Part model, mm, in its own coordinate system. A direction names the side the tool comes from. Round coordinates to 2 decimals unless told otherwise and drop trailing zeros. Loops run counter-clockwise (first coordinate to the right, second up) from the corner with the lowest first, then second, coordinate; pieces in that order, holes last. Notation, with made-up numbers: (-13.5, 86) -> (38.5, 86) arc R7 cw to (38.5, 98) -> close; hole circle Ø7 at (67.5, -32.5). An arc over 180 degrees is marked (long way). Answer as a JSON object with one key per item and string values. Group by question number.
from build123d import *

# Parameters (mm, degrees)
SKETCH1_W      = 50.1
SKETCH1_H      = 28.1
SKETCH1_R      = 1.7
EXTRUDE1_DEPTH = 1.54
SKETCH2_W      = 2.56
SKETCH2_H      = 15.1
SKETCH2_W_2    = 7.7
SKETCH2_H_2    = 5.4
EXTRUDE3_DEPTH = 8.4
SKETCH3_W      = 5.9
SKETCH3_H      = 7.94
EXTRUDE4_DEPTH = 5.15


with BuildPart() as part:
    # Sketch1 → Extrude1 (new body)
    with BuildSketch(Plane(origin=(0, 0, 0), x_dir=(1, 0, 0), z_dir=(0, 1, 0))):
        with Locations((-74.07266419, 15.871623192)):
            Rectangle(SKETCH1_W, SKETCH1_H)
        with Locations(Location((-96.42266419, 27.221623192, 0), (0, 0, 270))):
            Circle(SKETCH1_R, mode=Mode.SUBTRACT)
        with Locations(Location((-51.72266419, 27.221623192, 0), (0, 0, 90))):
            Circle(SKETCH1_R, mode=Mode.SUBTRACT)
        with Locations(Location((-51.72266419, 4.521623192, 0), (0, 0, 270))):
            Circle(SKETCH1_R, mode=Mode.SUBTRACT)
        with Locations(Location((-96.42266419, 4.521623192, 0), (0, 0, 90))):
            Circle(SKETCH1_R, mode=Mode.SUBTRACT)
    extrude(amount=EXTRUDE1_DEPTH)

    # Sketch2 → Extrude3 (add)
    with BuildSketch(Plane(origin=(0, 1.54, 0), x_dir=(1, 0, 0), z_dir=(0, 1, 0))):
        with Locations((-50.30266419, 15.871623192)):
            Rectangle(SKETCH2_W, SKETCH2_H)
        with Locations((-70.52266419, 4.521623192)):
            Rectangle(SKETCH2_W_2, SKETCH2_H_2)
    extrude(amount=EXTRUDE3_DEPTH)

    # Sketch3 → Extrude4 (add)
    with BuildSketch(Plane(origin=(0, 1.54, 0), x_dir=(1, 0, 0), z_dir=(0, 1, 0))):
        with Locations((-96.17266419, 19.101623192)):
            Rectangle(SKETCH3_W, SKETCH3_H)
    extrude(amount=EXTRUDE4_DEPTH)


solid = part.part
Item 1: Which spindle directions (+Z, -Z, +X, -X, +Y, -Y) get a long thin tool onto all of the face, cutting with end or side? Do faces 1 (the face through (-74.373, 6, -4)), 2 (the face through (-93.223, 4, -19)), 3 (the face through (-96, 4, -15.132)), 4 (the face through (-96, 4, -23.072)). Say none if no direction does.
Item 2: Two-plate mould, pull along Z, no slides. Class faces 5 (the face through (-50, 9.94, -16)), 6 (the face through (-97.931, 0.759, -26.437)), 7 (the face through (-74, 1, -29.922)): pulls with the +Z half, pulls with the -Z half, needs draft (parallel to the pull), parting line crosses it, or undercut.
Item 3: Band-saw the part on C-C, the plane y = 9. List the corners of the cut face in (x, z).
Item 4: Band-saw the part on B-B, the plane z = -28. List the corners of the cut face in (x, y).
Item 5: Band-saw the part on D-D, the plane x = -68.5. List the corners of the cut face in (y, z), plus the area to 3 significant figures.
Item 6: Drop flat-ended pins along their axis: pin 1 Ø2.5 at (x, z) = (-96.42, -27.22) entering from +Y; pin 2 Ø0.8 at (x, y) = (-50, 4) entering from +Z; pin 3 Ø5.5 at (x, y) = (-95.5, 5) entering from -Z; pin 4 Ø4 at (x, z) = (-51.72, -27.22) entering from +Y. Give the stop position or say it passes through.
Item 7: Band-saw the part on A-A, the plane y = 5.5. List the corners of the cut face in (x, z), plus the area to 3 significant figures.
Item 8: Drill centre lines: line 1 (X direction, y = 5, z = -17.5); line 2 (X direction, y = 7.75, z = -13); line 3 (Y direction, x = -76.5, z = -7). Where is each one in solid material? Low to high.
Entries:
{
 "1": {"face 1": "+Z, -Z, -X, +Y", "face 2": "+Z, -Z, +Y", "face 3": "+Z, -X, +Y", "face 4": "-Z, -X, +Y"},
 "2": {"face 5": "needs draft", "face 6": "undercut", "face 7": "pulls with the -Z half"},
 "3": {"outline": "(-74.37, -7.22) -> (-66.67, -7.22) -> (-66.67, -1.82) -> (-74.37, -1.82) -> close; (-51.58, -23.42) -> (-49.02, -23.42) -> (-49.02, -8.32) -> (-51.58, -8.32) -> close"},
 "4": {"outline": "(-99.12, 0) -> (-97.93, 0) -> (-97.93, 1.54) -> (-99.12, 1.54) -> close; (-94.91, 0) -> (-53.23, 0) -> (-53.23, 1.54) -> (-94.91, 1.54) -> close; (-50.21, 0) -> (-49.02, 0) -> (-49.02, 1.54) -> (-50.21, 1.54) -> close"},
 "5": {"outline": "(0, -29.92) -> (1.54, -29.92) -> (1.54, -7.22) -> (9.94, -7.22) -> (9.94, -1.82) -> (0, -1.82) -> close", "area": "88.6 mm²"},
 "6": {"pin 1": "through", "pin 2": "z = -8.32", "pin 3": "z = -23.07", "pin 4": "y = 1.54"},
 "7": {"outline": "(-99.12, -23.07) -> (-93.22, -23.07) -> (-93.22, -15.13) -> (-99.12, -15.13) -> close; (-74.37, -7.22) -> (-66.67, -7.22) -> (-66.67, -1.82) -> (-74.37, -1.82) -> close; (-51.58, -23.42) -> (-49.02, -23.42) -> (-49.02, -8.32) -> (-51.58, -8.32) -> close", "area": "127 mm²"},
 "8": {"line 1": "-99.12 to -93.22, -51.58 to -49.02", "line 2": "-51.58 to -49.02", "line 3": "0 to 1.54"}
}
